from build123d import *

# Parameters (mm, degrees)
BOSS_EXTRUDE1_DEPTH = 3
SKETCH2_R           = 1.65
CUT_EXTRUDE1_DEPTH  = 4
SKETCH3_W           = 30
SKETCH3_H           = 3
BOSS_EXTRUDE2_DEPTH = 8
BOSS_EXTRUDE3_DEPTH = 30
BOSS_EXTRUDE4_DEPTH = 3


with BuildPart() as part:
    # Sketch1 → Boss-Extrude1 (new body)
    with BuildSketch(Plane(origin=(0, 0, 0), x_dir=(1, 0, 0), z_dir=(0, 1, 0))):
        Polygon((15, -28), (15, 30), (-15, 30), (-15, -28), (-15, -31), (15, -31), align=None)
    extrude(amount=BOSS_EXTRUDE1_DEPTH)

    # Sketch2 → Cut-Extrude1 (cut)
    with BuildSketch(Plane(origin=(0, 3, 0), x_dir=(1, 0, 0), z_dir=(0, 1, 0))):
        with Locations((-7, 25.5)):
            Circle(SKETCH2_R)
        with Locations((7, 25.5)):
            Circle(SKETCH2_R)
        with Locations((-7, 9.5)):
            Circle(SKETCH2_R)
        with Locations((7, 9.5)):
            Circle(SKETCH2_R)
    extrude(amount=-CUT_EXTRUDE1_DEPTH, mode=Mode.SUBTRACT)

    # Sketch3 → Boss-Extrude2 (add)
    with BuildSketch(Plane.XY.offset(31)):
        with Locations((0, 1.5)):
            Rectangle(SKETCH3_W, SKETCH3_H)
    extrude(amount=BOSS_EXTRUDE2_DEPTH)

    # Sketch5 → Boss-Extrude3 (add)
    with BuildSketch(Plane.ZY.offset(15)):
        Polygon((39, 0), (8.218187101, -84.572335871), (5.399109238, -83.546275441), (35.807466683, 0), align=None)
    extrude(amount=-BOSS_EXTRUDE3_DEPTH)

    # Sketch6 → Boss-Extrude4 (add)
    with BuildSketch(Plane(origin=(15, 0, 0), x_dir=(0, 0, -1), z_dir=(1, 0, 0))):
        Polygon((30, 0), (-5.399109238, -83.546275441), (-8.218187101, -84.572335871), (-39, 0), (-39, 3), (30, 3), align=None)
    extrude(amount=-BOSS_EXTRUDE4_DEPTH)


solid = part.part
Model file for the job. Use its own axes, mm. A direction names the side the tool comes from. Give positions to 0.01 mm unless a question says otherwise; leave off trailing zeros. Order: outer loops, then holes, each group sorted by start corner. A loop starts at its lowest first (then second) coordinate and runs counter-clockwise, first axis right, second up. Notation, with made-up numbers: M 60.25,1 L 101.25,1 A13 ccw 101.25,25 Z; hole C 82,13 d8. An arc over 180 degrees is marked long. Write item = value, one per line.
Q1. Cut at B-B, the plane z = -25.5. List the corners of the cut face in (x, y), then the cut area to 3 significant figures.
Derived:
outline = M -15,0 L -8.65,0 L -8.65,3 L -15,3 Z; M -5.35,0 L 5.35,0 L 5.35,3 L -5.35,3 Z; M 8.65,0 L 12,0 L 12,-10.62 L 15,-10.62 L 15,3 L 8.65,3 Z
area = 102 mm2
Q2. Two-plate mould, pull along Z, no slides. Class faces 1 (the cylindrical face through (-8.31, 1.52, -8.5)), 2 (the flat face through (-1.69, -42.36, 20.39)), 3 (the flat face through (15, -30, 4)), 4 (the cylindrical face through (5.69, 1.52, -8.5)): pulls with the +Z half, pulls with the -Z half, needs draft (parallel to the pull), parting line crosses it, or undercut.
Derived:
face_1 = undercut
face_2 = pulls with the -Z half
face_3 = needs draft
face_4 = undercut
Q3. Cut at A-A, the plane x = 7. List the corners of the cut face in (y, z).
Derived:
outline = M -84.57,8.22 L -83.55,5.4 L 0,35.81 L 0,-7.85 L 3,-7.85 L 3,39 L 0,39 Z; M 0,-30 L 3,-30 L 3,-27.15 L 0,-27.15 Z; M 0,-23.85 L 3,-23.85 L 3,-11.15 L 0,-11.15 Z
Q4. Cut at D-D, the plane z = 34.5. List the corners of the cut face in (x, y).
Derived:
outline = M -15,-12.36 L 15,-12.36 L 15,3 L -15,3 L -15,0 L 12,0 L 12,-3.59 L -15,-3.59 Z
Q5. Drill centre lines: line 1 (X direction, y = 1.85, z = -25.5); line 2 (Z direction, x = -7, y = 2.1); line 3 (X direction, y = -0.5, z = 5). Where is each one in solid material? Low to high. Write a range as [from, to].
Derived:
line_1 = [-15, -8.65], [-5.35, 5.35], [8.65, 15]
line_2 = [-30, -27.15], [-23.85, -11.15], [-7.85, 39]
line_3 = [12, 15]
Q6. Cut at C-C, the plane y = -41. List the corners of the cut face in (x, z).
Derived:
outline = M -15,20.88 L 12,20.88 L 12,-12.63 L 15,-12.63 L 15,24.08 L -15,24.08 Z
Q7. Flat gauge pins, fed straight in: pin 1 (6 mm diameter, centred on x = -7.5, y = -20, fed in from +Z); pin 2 (4.5 mm diameter, centred on x = 7, z = -9.5, fed in from -Y); pin 3 (8 mm diameter, centred on x = 5, z = 12, fed in from -Y); pin 4 (2 mm diameter, centred on x = -7, z = -9.5, fed in from -Y). Where does each tip first touch, or does it go through?
Derived:
pin_1 = 32.81
pin_2 = 0
pin_3 = -84.57
pin_4 = through
Q8. Tool access for faces 5 (the flat face through (-0.21, -84.066, 6.828)), 6 (the flat face through (12, -23, 2)): list every direction of +Z, -Z, +X, -X, +Y, -Y with a clear straight run to the whole face (end or side of a thin tool).
Derived:
face_5 = -Z, +X, -X, -Y
face_6 = -Z, -X
